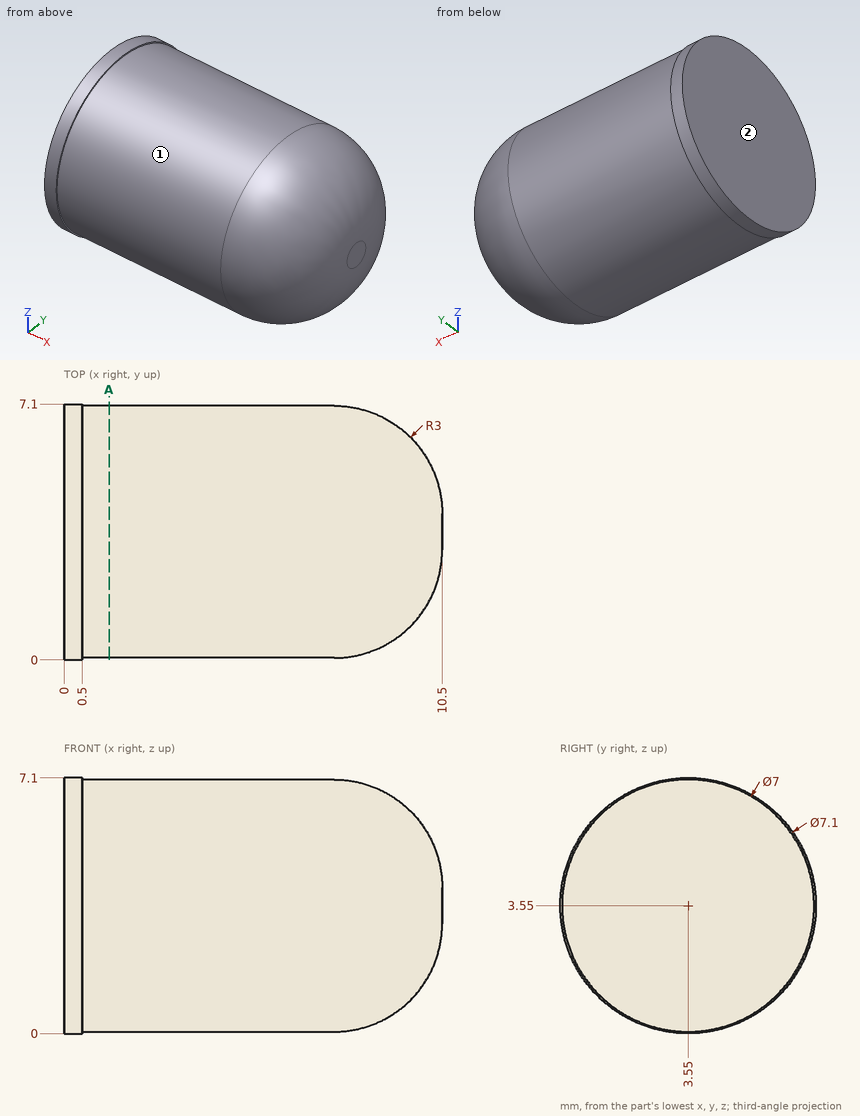
The figure shows three views and two pictorial views of one solid part (mm, origin at its lowest corner). Answer the questions. A direction names the side the tool comes from. Round coordinates to 2 decimals unless told otherwise and drop trailing zeros. Loops run counter-clockwise (first coordinate to the right, second up) from the corner with the lowest first, then second, coordinate; pieces in that order, holes last. Notation, with made-up numbers: (-8.5, 12.5) -> (43.5, 12.5) arc R21 ccw to (43.5, 37.5) -> close; hole circle Ø2 at (88.5, 61). An arc over 180 degrees is marked (long way). Use one line per item in the form item = value.
(1) Flat-ended cylindrical pins translate along their axes: P1, Ø4, axis at x = 4, y = 3.5, coming from the +Z side; P2, Ø3, axis at x = 7.5, z = 2, coming from the -Y side. Find the tip coordinate at first contact, or state that the pin passes through.
Answer list:
P1 = 7.05
P2 = 0.05
(2) A tool of negligible diameter and unlimited length cuts with its end or side. For the marked faces 1 and 2, from which of +Z, -Z, +X, -X, +Y, -Y can it reach the whole face along a straight path? Write none if from no direction.
Answer list:
face_1 = +X
face_2 = +Z, -Z, -X, +Y, -Y
(3) Find section A-A on x = 1.25. Give the vertices of the cut face in (y, z), then the cut area to 3 significant figures.
Answer list:
outline = circle Ø7 at (3.55, 3.55)
area = 38.5 mm2
(4) Straight lines are drawn through the part: line 1 (X direction, y = 3.75, z = 3); line 2 (Y direction, x = 2.25, z = 3.5); line 3 (Z direction, x = 3.5, y = 0.75). For each, find the intervals that lie inside material, in ascending order.
Answer list:
line_1 = 0 to 10.5
line_2 = 0.05 to 7.05
line_3 = 1.45 to 5.65
